Verification items for the finished model (mm, model axes). Round coordinates to 2 decimals unless told otherwise and drop trailing zeros. Order: outer loops, then holes, each group sorted by start corner. A loop starts at its lowest first (then second) coordinate and runs counter-clockwise, first axis right, second up. Notation, with made-up numbers: (-12, 52) -> (25, 52) arc R9 ccw to (25, 59) -> close; hole circle Ø8 at (-17.75, 49.5). An arc over 180 degrees is marked (long way). Write item = value, one per line. Start each with the question number.
from build123d import *

# Parameters (mm, degrees)
CHAMFER_1_SIZE      = 0.5
SKETCH_2_R          = 2
CUT_EXTRUDE_1_DEPTH = 9


with BuildPart() as part:
    # 草图1 → 旋转1 (revolve)
    with BuildSketch(Plane.XY, mode=Mode.PRIVATE) as revolve_1_sk:
        Polygon((-89, 0), (89, 0), (89, 4), (87.5, 4), (87.5, 3.5), (86.5, 3.5), (86.5, 4), (80.5, 4), (80.5, 3.5), (79.5, 3.5), (79.5, 4), (-79.5, 4), (-79.5, 3.5), (-80.5, 3.5), (-80.5, 4), (-86.5, 4), (-86.5, 3.5), (-87.5, 3.5), (-87.5, 4), (-89, 4), align=None)
    revolve(revolve_1_sk.sketch.rotate(Axis((25.510334062, 0, 0), (1, 0, 0)), 90), axis=Axis((25.510334062, 0, 0), (1, 0, 0)))

    # 倒角1
    chamfer_1_edges = [part.edges().sort_by_distance(p)[0] for p in [
        (89, 0, -4),
        (-89, 0, -4),
    ]]
    chamfer(chamfer_1_edges, length=CHAMFER_1_SIZE)

    # 草图2 → 切除-拉伸1 (cut)
    with BuildSketch(Plane.XY.offset(5)):
        with Locations((43, 0)):
            Circle(SKETCH_2_R)
        with Locations((-43, 0)):
            Circle(SKETCH_2_R)
    extrude(amount=-CUT_EXTRUDE_1_DEPTH, mode=Mode.SUBTRACT)


solid = part.part
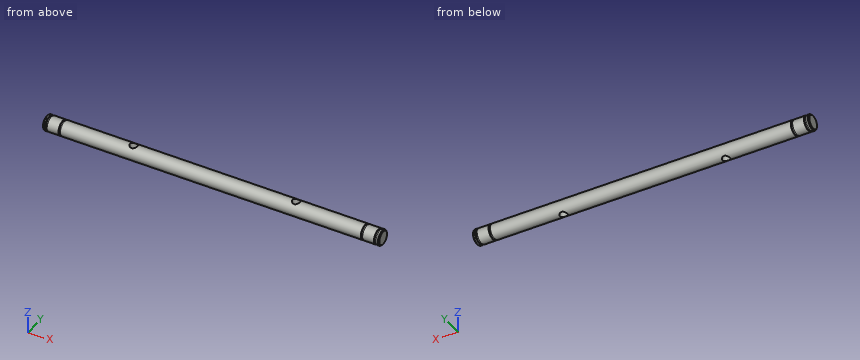
(1) Scan lines: line 1 along X through (y, z) = (-3.5, 0.5); line 2 along X through (y, z) = (0, 2.25); line 3 along X through (y, z) = (0.5, -3). Record each from-to range of solid material in increasing order. Write a range as from..to.
(2) Depth check by flat-ended pin: pin 1 (2 mm diameter, centred on x = -34, z = 1.5, fed in from +Y); pin 2 (2 mm diameter, centred on x = 44, y = -2.5, fed in from +Z). Enter the tip coordinate at first touch or a pass-through.
(3) Cross-section at A-A (y = 0). Give the number of separate pieces and of enclosed holes in the cut face, and give its area (3 significant figures).
(4) Cross-section at D-D (x = 71). Enter the section's corners in (y, z).
(5) Cross-section at C-C (x = -43). Enter the section's corners in (y, z), and give its area (3 significant figures).
Outcome:
q1.line_1 = -88.96..-87.5, -86.5..-80.5, -79.5..79.5, 80.5..86.5, 87.5..88.96
q1.line_2 = -89..-45, -41..41, 45..89
q1.line_3 = -89..-44.94, -41.06..41.06, 44.94..89
q2.pin_1 = 3.97
q2.pin_2 = 3.69
q3.separate_pieces = 3
q3.enclosed_holes = 0
q3.area = 1,360 mm^2
q4.outline = circle Ø8 at (0, 0)
q5.outline = (-2, -3.46) -> (-2, 3.46) arc R4 ccw to start; (2, -3.46) arc R4 ccw to (2, 3.46) -> close
q5.area = 19.7 mm^2
